Work out the finished part from the listing and answer in its coordinate system (mm). A direction names the side the tool comes from. Coordinates: 2 decimals unless noted, no trailing zeros. Order: outer loops, then holes, each group sorted by start corner. A loop starts at its lowest first (then second) coordinate and runs counter-clockwise, first axis right, second up. Notation, with made-up numbers: M 72.25,-37.5 L 127.25,-37.5 A12 ccw 127.25,-20.5 Z; hole C 20,-19 d7. An arc over 180 degrees is marked long. Answer in a Markdown table with one row per item. Add a question column.
Item 1: The part is cut by section B-B (x = 0). Write down the section's boundary in (y, z), then the cut area to 3 significant figures.
Item 2: The part is cut by section D-D (y = 5.5). Write down the section's boundary in (x, z).
Item 3: Which of the six approach directions +Z, -Z, +X, -X, +Y, -Y give full straight-line access (tool end or side, diameter ignored) to faces 1 (the face through (-0.01, 5.07, 1.12)), 2 (the face through (-3, 3.5, 6)), 3 (the face through (0, 10, 2))?
Item 4: The part is cut by section C-C (y = 1). Write down the section's boundary in (x, z), then the cut area to 3 significant figures.
Item 5: The part is cut by section A-A (z = 0). Write down the section's boundary in (x, y).
Item 6: Consider line 1 (X direction, y = 8.75, z = -2.25) (1 decimal); line 2 (Y direction, x = 2.75, z = -9.75); line 3 (X direction, y = 5, z = 2.75) (3 decimals). Determine where each line is inside the solid, lowest interval first. Write a range as from..to.
Item 7: The mould has two halves that part along Z. Classify faces 4 (the face through (0, 0, -3)), 5 (the face through (12.447, 1.479, 2.764)), 6 (the face through (0.8, 5.1, 2.1)): released by +Z, released by -Z, zero draft, split by the parting line, or undercut.
Item 8: Flat-ended cylindrical pins translate along their axes: pin 1 Ø3 at (x, y) = (2, 2) entering from -Z; pin 2 Ø1 at (y, z) = (1.5, 9) entering from +X; pin 3 Ø1.5 at (y, z) = (3.5, -3.5) entering from -X. Find the tip coordinate at first contact, or state that the pin passes through.
from build123d import *

# Parameters (mm, degrees)
SKETCH1_R           = 12.75
BOSS_EXTRUDE2_DEPTH = 3.5
SKETCH2_R           = 5.75
BOSS_EXTRUDE3_DEPTH = 6.5
CUT_EXTRUDE1_DEPTH  = 10
FILLET3_R           = 0.5
FILLET4_R           = 0.5


with BuildPart() as part:
    # Sketch1 → Boss-Extrude2 (new body)
    with BuildSketch(Plane(origin=(0, 0, 0), x_dir=(1, 0, 0), z_dir=(0, 1, 0))):
        with Locations(Location((0, 0, 0), (0, 0, 90))):
            Circle(SKETCH1_R)
    extrude(amount=BOSS_EXTRUDE2_DEPTH)

    # Sketch2 → Boss-Extrude3 (add)
    with BuildSketch(Plane(origin=(0, 3.5, 0), x_dir=(1, 0, 0), z_dir=(0, 1, 0))):
        with Locations(Location((0, 0, 0), (0, 0, 270))):
            Circle(SKETCH2_R)
    extrude(amount=BOSS_EXTRUDE3_DEPTH)

    # Sketch3 → Cut-Extrude1 (cut)
    with BuildSketch(Plane(origin=(0, 10, 0), x_dir=(1, 0, 0), z_dir=(0, 1, 0))):
        with BuildLine():
            Line((-0.447213595, 1.394427191), (-1.135934639, 2.771869278))
            ThreePointArc((-1.135934639, 2.771869278), (-1.447076632, 3.029390861), (-1.847006274, 2.972972894))
            ThreePointArc((-1.847006274, 2.972972894), (-3.5, 0), (-1.847006274, -2.972972894))
            ThreePointArc((-1.847006274, -2.972972894), (-1.447076632, -3.029390861), (-1.135934639, -2.771869278))
            Line((-1.135934639, -2.771869278), (-0.447213595, -1.394427191))
            ThreePointArc((-0.447213595, -1.394427191), (0, -1.118033989), (0.447213595, -1.394427191))
            Line((0.447213595, -1.394427191), (1.135934639, -2.771869278))
            ThreePointArc((1.135934639, -2.771869278), (1.447076632, -3.029390861), (1.847006274, -2.972972894))
            ThreePointArc((1.847006274, -2.972972894), (3.5, 0), (1.847006274, 2.972972894))
            ThreePointArc((1.847006274, 2.972972894), (1.447076632, 3.029390861), (1.135934639, 2.771869278))
            Line((1.135934639, 2.771869278), (0.447213595, 1.394427191))
            ThreePointArc((0.447213595, 1.394427191), (0, 1.118033989), (-0.447213595, 1.394427191))
        make_face()
    extrude(amount=-CUT_EXTRUDE1_DEPTH, mode=Mode.SUBTRACT)

    # Fillet3
    fillet3_edges = [part.edges().sort_by_distance(p)[0] for p in [
        (0, 3.5, 12.75),
        (0, 3.5, -5.75),
    ]]
    fillet(fillet3_edges, radius=FILLET3_R)

    # Fillet4
    fillet4_edges = [part.edges().sort_by_distance(p)[0] for p in [
        (0, 10, -5.75),
    ]]
    fillet(fillet4_edges, radius=FILLET4_R)


solid = part.part
Reply:
| question | item | result |
|---|---|---|
| 1 | outline | M 0,-12.75 L 3,-12.75 A0.5 ccw 3.5,-12.25 L 3.5,-6.25 A0.5 cw 4,-5.75 L 9.5,-5.75 A0.5 ccw 10,-5.25 L 10,-1.12 L 0,-1.12 Z; M 0,1.12 L 10,1.12 L 10,5.25 A0.5 ccw 9.5,5.75 L 4,5.75 A0.5 cw 3.5,6.25 L 3.5,12.25 A0.5 ccw 3,12.75 L 0,12.75 Z |
| 1 | area | 142 mm2 |
| 2 | outline | C 0,0 d11.5; hole M -1.85,-2.97 A0.5 ccw -1.14,-2.77 L -0.45,-1.39 A0.5 cw 0.45,-1.39 L 1.14,-2.77 A0.5 ccw 1.85,-2.97 A3.5 ccw 1.85,2.97 A0.5 ccw 1.14,2.77 L 0.45,1.39 A0.5 cw -0.45,1.39 L -1.14,2.77 A0.5 ccw -1.85,2.97 A3.5 ccw Z |
| 3 | face 1 | +Y, -Y |
| 3 | face 2 | +Y |
| 3 | face 3 | +Z, -Z, +X, -X, +Y |
| 4 | outline | C 0,0 d25.5; hole M -1.85,-2.97 A0.5 ccw -1.14,-2.77 L -0.45,-1.39 A0.5 cw 0.45,-1.39 L 1.14,-2.77 A0.5 ccw 1.85,-2.97 A3.5 ccw 1.85,2.97 A0.5 ccw 1.14,2.77 L 0.45,1.39 A0.5 cw -0.45,1.39 L -1.14,2.77 A0.5 ccw -1.85,2.97 A3.5 ccw Z |
| 4 | area | 480 mm2 |
| 5 | outline | M -12.75,0 L -3.5,0 L -3.5,10 L -5.25,10 A0.5 ccw -5.75,9.5 L -5.75,4 A0.5 cw -6.25,3.5 L -12.25,3.5 A0.5 ccw -12.75,3 Z; M 3.5,0 L 12.75,0 L 12.75,3 A0.5 ccw 12.25,3.5 L 6.25,3.5 A0.5 cw 5.75,4 L 5.75,9.5 A0.5 ccw 5.25,10 L 3.5,10 Z |
| 6 | line 1 | x = -5.3..-2.7, -0.9..0.9, 2.7..5.3 |
| 6 | line 2 | y = 0..3.5 |
| 6 | line 3 | x = -5.05..-2.165, -1.125..1.125, 2.165..5.05 |
| 7 | face 4 | zero draft |
| 7 | face 5 | split by the parting line |
| 7 | face 6 | undercut |
| 8 | pin 1 | stops at z = -12.74 |
| 8 | pin 2 | stops at x = 9.5 |
| 8 | pin 3 | stops at x = -12.41 |
